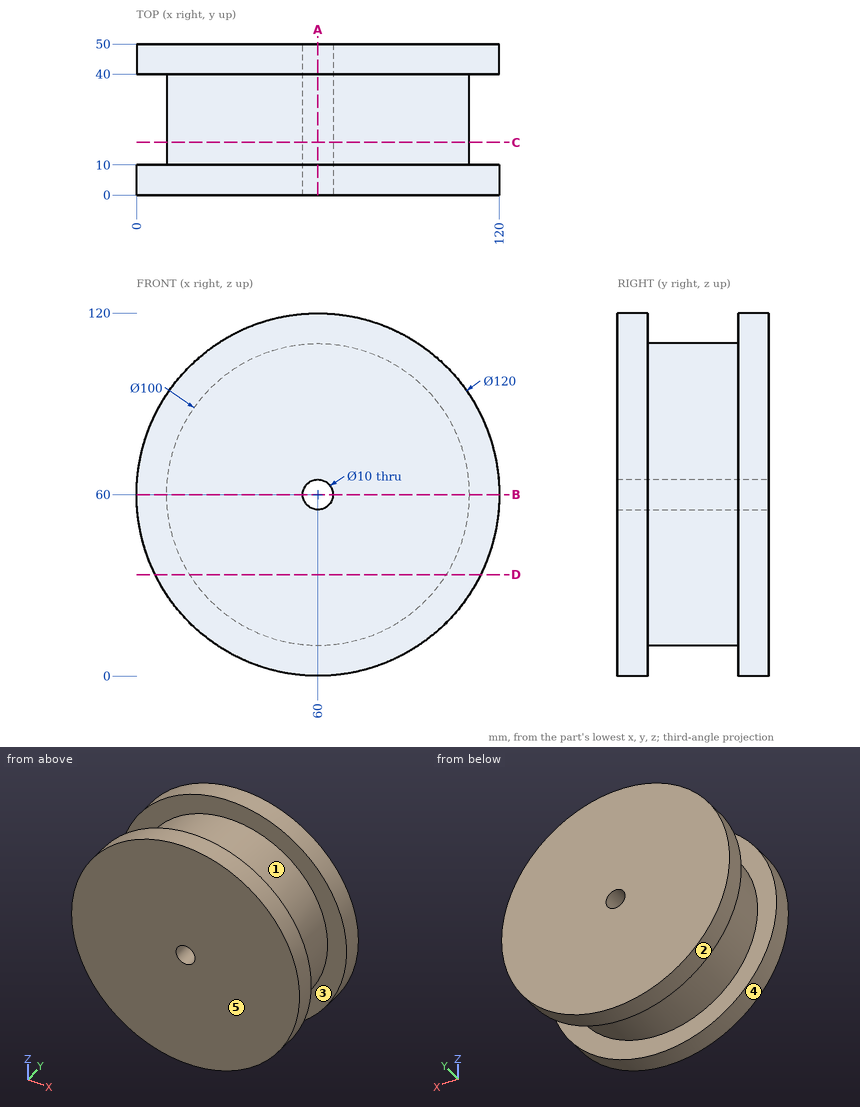
Input: dimensioned drawing with shaded views. Units: mm. Origin: part minimum x, y, z. A direction names the side the tool comes from. Coordinates: 2 decimals unless noted, no trailing zeros. Order: outer loops, then holes, each group sorted by start corner. A loop starts at its lowest first (then second) coordinate and runs counter-clockwise, first axis right, second up. Notation, with made-up numbers: (45, 54.5) - (85, 54.5) arc R29 cw to (85, 83.5) - close; hole circle Ø4 at (43.5, 75.25). An arc over 180 degrees is marked (long way). Put each result on its own line as item: value.
1. Draft query along Y for the marked faces 3, 4 and 5. Return one class per face: pulls with the +Y half, pulls with the -Y half, needs draft (parallel to the pull), parting line crosses it, or undercut.
Report:
face 3: undercut
face 4: needs draft
face 5: pulls with the -Y half
2. Reachability of the marked faces 1 and 2 from +Z, -Z, +X, -X, +Y, -Y: full face, straight path, thin tool, end or side. Return the list, or none.
Report:
face 1: none
face 2: +Y, -Y
3. Contact query for flat-ended pins moving along their axis: pin 1 Ø10 at (y, z) = (11, 75.5) entering from +X; pin 2 Ø5 at (x, y) = (36.5, 20.5) entering from -Z; pin 3 Ø5 at (x, z) = (69.5, 31.5) entering from -Y; pin 4 Ø12 at (x, y) = (14.5, 31.5) entering from -Z. Output: stop coordinate, or through.
Report:
pin 1: stops at x = 119.06
pin 2: stops at z = 14.62
pin 3: stops at y = 0
pin 4: stops at z = 29.34
4. Line query: line 1 along Z through (x, y) = (60, 36.5); line 2 along Y through (x, z) = (5, 72.5). Output: solid intervals per line, ascending.
Report:
line 1: z = 10 to 55, 65 to 110
line 2: y = 0 to 10, 40 to 50
5. Cut plane C-C on y = 17.5. Return the cut outline in (x, z), then the cut area to 3 significant figures.
Report:
outline: circle Ø100 at (60, 60); hole circle Ø10 at (60, 60)
area: 7,780 mm2
6. Cut plane D-D on z = 33.5. Return the cut outline in (x, y), then the cut area to 3 significant figures.
Report:
outline: (6.17, 0) - (113.83, 0) - (113.83, 10) - (102.4, 10) - (102.4, 40) - (113.83, 40) - (113.83, 50) - (6.17, 50) - (6.17, 40) - (17.6, 40) - (17.6, 10) - (6.17, 10) - close
area: 4,700 mm2
7. Cut plane A-A on x = 60. Return the cut outline in (y, z), then the cut area to 3 significant figures.
Report:
outline: (0, 0) - (10, 0) - (10, 10) - (40, 10) - (40, 0) - (50, 0) - (50, 55) - (0, 55) - close; (0, 65) - (50, 65) - (50, 120) - (40, 120) - (40, 110) - (10, 110) - (10, 120) - (0, 120) - close
area: 4,900 mm2
8. Cut plane B-B on z = 60. Return the cut outline in (x, y).
Report:
outline: (0, 0) - (55, 0) - (55, 50) - (0, 50) - (0, 40) - (10, 40) - (10, 10) - (0, 10) - close; (65, 0) - (120, 0) - (120, 10) - (110, 10) - (110, 40) - (120, 40) - (120, 50) - (65, 50) - close
